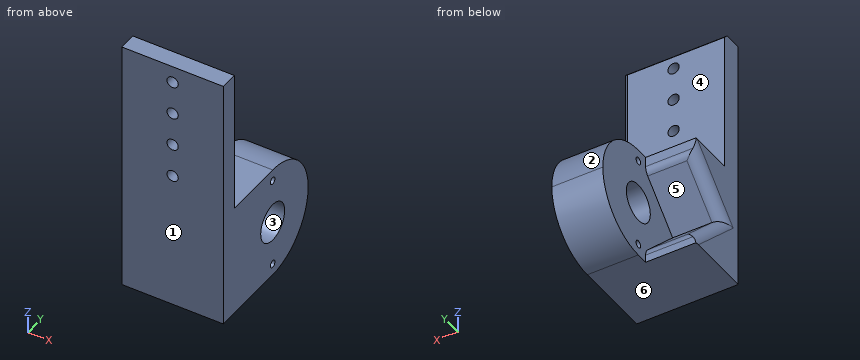
from build123d import *

# Parameters (mm, degrees)
SKETCH1_W           = 57.15
SKETCH1_H           = 145.034
BOSS_EXTRUDE1_DEPTH = 25.4
SKETCH4_R           = 3.175
CUT_EXTRUDE3_DEPTH  = 158.943482474
SKETCH7_W           = 28.702
SKETCH7_H           = 64.008
BOSS_EXTRUDE2_DEPTH = 76.454
FILLET1_R           = 32.004
SKETCH9_R           = 10.795
SKETCH9_R_2         = 2.032
CUT_EXTRUDE5_DEPTH  = 76.454
CUT_EXTRUDE7_DEPTH  = 12.954
CHAMFER1_SIZE       = 2.54
BOSS_EXTRUDE4_DEPTH = 28.448
FILLET3_R           = 6.35


# Some blends are built 0.0001 mm under size
with BuildPart() as part:
    # Sketch1 → Boss-Extrude1 (new body)
    with BuildSketch(Plane(origin=(0, 0, 0), x_dir=(1, 0, 0), z_dir=(0, 1, 0))):
        with Locations((28.575, 72.517)):
            Rectangle(SKETCH1_W, SKETCH1_H)
    extrude(amount=BOSS_EXTRUDE1_DEPTH)

    # Sketch4 → Cut-Extrude3 (cut, through all)
    with BuildSketch(Plane(origin=(0, 0, 0), x_dir=(-1, 0, 0), z_dir=(0, -1, 0))):
        with Locations(Location((-28.575, 9.525, 0), (0, 0, 90))):
            Circle(SKETCH4_R)
        with Locations(Location((-28.575, 28.575, 0), (0, 0, 90))):
            Circle(SKETCH4_R)
        with Locations(Location((-28.575, 47.625, 0), (0, 0, 90))):
            Circle(SKETCH4_R)
        with Locations(Location((-28.575, 66.675, 0), (0, 0, 90))):
            Circle(SKETCH4_R)
    extrude(amount=-CUT_EXTRUDE3_DEPTH, mode=Mode.SUBTRACT)

    # Sketch7 → Boss-Extrude2 (add)
    with BuildSketch(Plane.XZ):
        with Locations((42.799, -113.03)):
            Rectangle(SKETCH7_W, SKETCH7_H)
    extrude(amount=-BOSS_EXTRUDE2_DEPTH)

    # Fillet1
    fillet1_edges = [part.edges().sort_by_distance(p)[0] for p in [
        (42.799, 76.454, -145.034),
        (42.799, 76.454, -81.026),
    ]]
    fillet(fillet1_edges, radius=FILLET1_R - 0.0001)  # a hair under: the kernel refuses the full size

    # Sketch9 → Cut-Extrude5 (cut)
    with BuildSketch(Plane.ZY.offset(-28.448)):
        with Locations((-113.03, 44.45)):
            Circle(SKETCH9_R)
        with Locations((-138.43, 44.45)):
            Circle(SKETCH9_R_2)
        with Locations((-87.63, 44.45)):
            Circle(SKETCH9_R_2)
    extrude(amount=-CUT_EXTRUDE5_DEPTH, mode=Mode.SUBTRACT)

    # Sketch10 → Cut-Extrude7 (cut)
    with BuildSketch(Plane(origin=(0, 25.4, 0), x_dir=(1, 0, 0), z_dir=(0, 1, 0))):
        Polygon((28.448, 113.03), (28.448, 81.026), (57.15, 81.026), (57.15, 0), (50.8, 0), (0, 0), (0, 113.03), (0, 145.034), (28.448, 145.034), align=None)
    extrude(amount=-CUT_EXTRUDE7_DEPTH, mode=Mode.SUBTRACT)

    # Chamfer1
    chamfer1_edges = [part.edges().sort_by_distance(p)[0] for p in [
        (57.15, 12.446, -40.513),
        (28.575, 12.446, 0),
    ]]
    chamfer(chamfer1_edges, length=CHAMFER1_SIZE)

    # Sketch14 → Boss-Extrude4 (add)
    with BuildSketch(Plane.ZY.offset(-28.448)):
        Polygon((-113.637411412, 13.462), (-138.021411412, 37.846), (-145.034, 37.846), (-145.034, 12.446), (-81.026, 12.446), (-81.026, 37.846), (-89.253411412, 37.846), align=None)
    extrude(amount=BOSS_EXTRUDE4_DEPTH)

    # Fillet3
    # the kernel refuses this fillet: 6.35 mm, written as the material it takes off along each edge
    with BuildSketch(Plane(origin=(0, 49.071320151, -78.028091261), x_dir=(1, 0, 0), z_dir=(0, -0.707106781186549, -0.7071067811865461)), Plane(origin=(0, 13.462, -113.637411412), x_dir=(1, 0, 0), z_dir=(0, 0.7071067811865438, -0.7071067811865512))) as fillet3_piece_1:
        with BuildLine():
            CenterArc((FILLET3_R, FILLET3_R), FILLET3_R, 180, 90)
            Line((0, FILLET3_R), (0, 0))
            Line((0, 0), (FILLET3_R, 0))
        make_face()
    extrude(amount=50.359183505, mode=Mode.SUBTRACT)
    with BuildSketch(Plane(origin=(28.448, 37.846, -89.253411412), x_dir=(0, -0.7071067811865475, -0.7071067811865475), z_dir=(-1, 0, 0)), Plane(origin=(28.448, 37.846, -138.021411412), x_dir=(0, 0, -1), z_dir=(-1, 0, 0))) as fillet3_piece_2:
        with BuildLine():
            CenterArc((FILLET3_R * 0.414213562373, FILLET3_R), FILLET3_R, 225, 45)
            Line((-FILLET3_R * 0.292893218813, FILLET3_R * 0.292893218813), (0, 0))
            Line((0, 0), (FILLET3_R * 0.414213562373, 0))
        make_face()
    extrude(amount=35.023640303, mode=Mode.SUBTRACT)
    with BuildSketch(Plane(origin=(0, 2.236679849, -102.412091261), x_dir=(1, 0, 0), z_dir=(0, 0.7071067811865438, -0.7071067811865512))) as fillet3_piece_3a_section:
        with BuildLine():
            CenterArc((FILLET3_R, FILLET3_R), FILLET3_R, 180, 90)
            Line((0, FILLET3_R), (0, 0))
            Line((0, 0), (FILLET3_R, 0))
        make_face()
    fillet3_piece_3a = extrude(amount=66.234183505, mode=Mode.PRIVATE)
    fillet3_piece_3a = split(fillet3_piece_3a, bisect_by=Plane(origin=(1.437608976, 12.445456945, -114.653954468), z_dir=(0, -0.7071067811865461, 0.707106781186549)), keep=Keep.TOP, mode=Mode.PRIVATE)
    with BuildSketch(Plane(origin=(0, 49.071320151, -78.028091261), x_dir=(1, 0, 0), z_dir=(0, -0.707106781186549, -0.7071067811865461))) as fillet3_piece_3b_section:
        with BuildLine():
            CenterArc((FILLET3_R, FILLET3_R), FILLET3_R, 180, 90)
            Line((0, FILLET3_R), (0, 0))
            Line((0, 0), (FILLET3_R, 0))
        make_face()
    fillet3_piece_3b = extrude(amount=66.234183505, mode=Mode.PRIVATE)
    fillet3_piece_3b = split(fillet3_piece_3b, bisect_by=Plane(origin=(1.437608976, 12.445456945, -112.620868357), z_dir=(0, -0.7071067811865512, -0.7071067811865438)), keep=Keep.TOP, mode=Mode.PRIVATE)
    fillet3_piece_3 = fillet3_piece_3a & fillet3_piece_3b
    add(fillet3_piece_3, mode=Mode.SUBTRACT)


solid = part.part
Check sheet for the modelled part. Datum: model origin and axes. Units: mm. Face numbers are marked on the shaded views. A direction names the side the tool comes from. Give positions to 0.01 mm unless a question says otherwise; leave off trailing zeros. Write each loop counter-clockwise with the first axis right and the second up, starting at its lowest first coordinate (ties: lowest second). Pieces come first, ordered by that corner, then holes. Notation, with made-up numbers: (-12.75, 76.25) -> (-2.75, 76.25) arc R23 ccw to (-2.75, 87.25) -> close; hole circle Ø4 at (41.25, 69). An arc over 180 degrees is marked (long way). Use one line per item in the form item = value. Start each with the question number.
1. Go/stop test with flat-tipped pins: P1, Ø3, axis at x = 49, z = -38, coming from the +Y side; P2, Ø6, axis at x = 15.5, z = -84, coming from the +Y side; P3, Ø6, axis at y = 13.5, z = -25, coming from the +X side. Record where each tip stops, or that it passes through.
2. Section check D-D (z = -39.5). Record the cut outline in (x, y), and give its area (3 significant figures).
3. Section check B-B (z = -66.5). Record the cut outline in (x, y), and give its area (3 significant figures).
4. Section check A-A (x = 46). Count the separate pieces of the cut face and the enclosed holes in it, and give its area (3 significant figures).
5. Section check C-C (x = 9). Record the cut outline in (y, z).
6. Mould release check, pull along Y, two halves, no side actions. Record for the marked faces 1, 2 and 3: pulls with the +Y half, pulls with the -Y half, needs draft (parallel to the pull), parting line crosses it, or undercut.
7. Access from +Z, -Z, +X, -X, +Y, -Y to the whole of each face (thin tool, end or side, straight path). Record for the marked faces 4, 5 and 6.
8. Thickness scan on line 1 along Z through (x, y) = (42, 44); line 2 along X through (y, z) = (46.5, -85); line 3 along Z through (x, y) = (38.5, 43). Record the ranges inside material, lowest first. Write a range as from..to.
Conclusion:
q1.P1 = 12.45
q1.P2 = 37.85
q1.P3 = 56.56
q2.outline = (0, 0) -> (57.15, 0) -> (57.15, 9.91) -> (54.61, 12.45) -> (0, 12.45) -> close
q2.area = 708 mm²
q3.outline = (0, 0) -> (25.4, 0) -> (25.4, 12.45) -> (0, 12.45) -> close; (31.75, 0) -> (57.15, 0) -> (57.15, 9.91) -> (54.61, 12.45) -> (31.75, 12.45) -> close
q3.area = 629 mm²
q4.separate_pieces = 1
q4.enclosed_holes = 3
q4.area = 5,070 mm²
q5.outline = (0, -145.03) -> (37.85, -145.03) -> (37.85, -140.65) arc R6.35 ccw to (35.99, -136.16) -> (13.46, -113.64) -> (35.99, -91.11) arc R6.35 ccw to (37.85, -86.62) -> (37.85, -81.03) -> (12.45, -81.03) -> (12.45, -2.54) -> (9.91, 0) -> (0, 0) -> close
q6.face_1 = pulls with the -Y half
q6.face_2 = pulls with the +Y half
q6.face_3 = undercut
q7.face_4 = +Z, +X, -X, +Y
q7.face_5 = -X, +Y
q7.face_6 = -Z, +X, -X, +Y, -Y
q8.line_1 = -145.03..-140.41, -136.45..-123.82, -102.24..-89.61, -85.65..-81.03
q8.line_2 = 28.45..57.15
q8.line_3 = -145.03..-139.85, -137.01..-123.73, -102.33..-89.05, -86.21..-81.03
